Check sheet for the modelled part. Datum: model origin and axes. Units: mm. Face numbers are marked on the shaded views. A direction names the side the tool comes from. Round coordinates to 2 decimals unless told otherwise and drop trailing zeros. Loops run counter-clockwise (first coordinate to the right, second up) from the corner with the lowest first, then second, coordinate; pieces in that order, holes last. Notation, with made-up numbers: M -14.5,-35 L 9.5,-35 A28 cw 9.5,-6 Z; hole C 42,70.5 d5. An arc over 180 degrees is marked long. Write item = value, one per line. Start each with the question number.
(1) Cross-section at C-C on z = -12.7. Record the boundary of the cut face in (x, y) (1 decimal).
(2) Cross-section at A-A on y = 12.7. Record the boundary of the cut face in (x, z) (1 decimal).
(3) Set-up check for the marked faces 1 and 2: record each of +Z, -Z, +X, -X, +Y, -Y from which the full face is reachable in a straight line by a thin tool's end or side.
(4) Cross-section at D-D on y = 116. Record the boundary of the cut face in (x, z), plus the area to 3 significant figures.
(5) Cross-section at B-B on x = 12.7. Record the boundary of the cut face in (y, z) (1 decimal), plus the area to 3 significant figures.
(6) Scan lines: L1, parallel to Y at x = -0.95, z = -12.7 (3 decimals); L2, parallel to Z at x = 3, y = 64; L3, parallel to X at y = 128, z = -22.25. Record each from-to range of solid material in increasing order. Write a range as from..to.
(7) Go/stop test with flat-tipped pins: P1, Ø8, axis at y = 118.5, z = -6.5, coming from the +X side; P2, Ø1, axis at x = 14.5, y = 127.5, coming from the -Z side; P3, Ø10, axis at y = 12.7, z = -12.7, coming from the -X side. Record where each tip stops, or that it passes through.
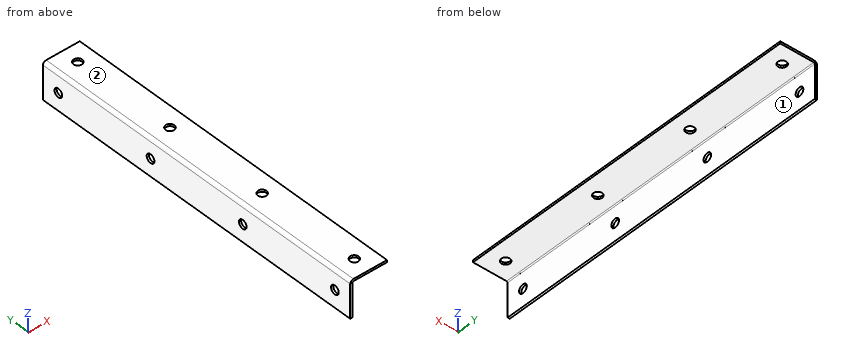
from build123d import *

# Parameters (mm, degrees)
BASE_FLANGE1_DEPTH = 254
SKETCH6_R          = 3.175
CUT_EXTRUDE1_DEPTH = 257.689472235
SKETCH7_R          = 3.175
CUT_EXTRUDE2_DEPTH = 257.689472235


# Sheet-metal steps are written as plain solids
with BuildPart() as part:
    # Sketch1 → Base-Flange1 (new body)
    with BuildSketch(Plane(origin=(0, 0, 0), x_dir=(1, 0, 0), z_dir=(0, 1, 0))):
        with BuildLine():
            Line((0, 25.4), (0, 0.7366))
            ThreePointArc((0, 0.7366), (0.215745145, 0.215745145), (0.7366, 0))
            Line((0.7366, 0), (25.4, 0))
            Line((25.4, 0), (25.4, -1.5875))
            Line((25.4, -1.5875), (0.7366, -1.5875))
            ThreePointArc((0.7366, -1.5875), (-0.90678687, -0.90678687), (-1.5875, 0.7366))
            Line((-1.5875, 0.7366), (-1.5875, 25.4))
            Line((-1.5875, 25.4), (0, 25.4))
        make_face()
    extrude(amount=BASE_FLANGE1_DEPTH)

    # Sketch6 → Cut-Extrude1 (cut, through all)
    with BuildSketch(Plane.XY.offset(1.5875)):
        with Locations((12.7, 241.3)):
            Circle(SKETCH6_R)
        with Locations((12.7, 165.1)):
            Circle(SKETCH6_R)
        with Locations((12.7, 88.9)):
            Circle(SKETCH6_R)
        with Locations((12.7, 12.7)):
            Circle(SKETCH6_R)
    extrude(amount=-CUT_EXTRUDE1_DEPTH, mode=Mode.SUBTRACT)

    # Sketch7 → Cut-Extrude2 (cut, through all)
    with BuildSketch(Plane.ZY.offset(1.5875)):
        with Locations((-12.7, 241.3)):
            Circle(SKETCH7_R)
        with Locations((-12.7, 165.1)):
            Circle(SKETCH7_R)
        with Locations((-12.7, 88.9)):
            Circle(SKETCH7_R)
        with Locations((-12.7, 12.7)):
            Circle(SKETCH7_R)
    extrude(amount=-CUT_EXTRUDE2_DEPTH, mode=Mode.SUBTRACT)


solid = part.part
Result:
q1.outline = M -1.6,0 L 0,0 L 0,9.5 L -1.6,9.5 Z; M -1.6,15.9 L 0,15.9 L 0,85.7 L -1.6,85.7 Z; M -1.6,92.1 L 0,92.1 L 0,161.9 L -1.6,161.9 Z; M -1.6,168.3 L 0,168.3 L 0,238.1 L -1.6,238.1 Z; M -1.6,244.5 L 0,244.5 L 0,254 L -1.6,254 Z
q2.outline = M -1.6,-25.4 L 0,-25.4 L 0,-15.9 L -1.6,-15.9 Z; M -1.6,-9.5 L 0,-9.5 L 0,-0.7 A0.7 cw 0.7,0 L 9.5,0 L 9.5,1.6 L 0.7,1.6 A2.3 ccw -1.6,-0.7 Z; M 15.9,0 L 25.4,0 L 25.4,1.6 L 15.9,1.6 Z
q3.face_1 = -Z, +X, +Y, -Y
q3.face_2 = +Z, +X, -X, +Y, -Y
q4.outline = M -1.59,-25.4 L 0,-25.4 L 0,-0.74 A0.74 cw 0.74,0 L 25.4,0 L 25.4,1.59 L 0.74,1.59 A2.32 ccw -1.59,-0.74 Z
q4.area = 82.1 mm^2
q5.outline = M 0,0 L 9.5,0 L 9.5,1.6 L 0,1.6 Z; M 15.9,0 L 85.7,0 L 85.7,1.6 L 15.9,1.6 Z; M 92.1,0 L 161.9,0 L 161.9,1.6 L 92.1,1.6 Z; M 168.3,0 L 238.1,0 L 238.1,1.6 L 168.3,1.6 Z; M 244.5,0 L 254,0 L 254,1.6 L 244.5,1.6 Z
q5.area = 363 mm^2
q6.L1 = 0..9.525, 15.875..85.725, 92.075..161.925, 168.275..238.125, 244.475..254
q6.L2 = 0..1.59
q6.L3 = -1.59..0
q7.P1 = 0
q7.P2 = 0
q7.P3 = -1.59
